```python
from build123d import *

# Parameters (mm, degrees)
BOSS_EXTRUDE1_DEPTH   = 6.35
F_4_40_TAPPED_HOLE1_D = 2.2606
SKETCH8_R             = 2.38125
CUT_EXTRUDE1_DEPTH    = 6.35
SKETCH9_R             = 1.4732
CUT_EXTRUDE2_DEPTH    = 14.088396137
SKETCH10_R            = 1.4732
CUT_EXTRUDE3_DEPTH    = 15.889903931
CHAMFER1_SIZE         = 1.778
CHAMFER1_SIZE_2       = 1.54559182


with BuildPart() as part:
    # Sketch1 → Boss-Extrude1 (new body)
    with BuildSketch(Plane(origin=(0, 0, 0), x_dir=(1, 0, 0), z_dir=(0, 1, 0))):
        with BuildLine():
            Line((-2.487063329, -0.254), (-9.521612731, -0.254))
            ThreePointArc((-9.521612731, -0.254), (0, -9.525), (9.521612731, -0.254))
            Line((9.521612731, -0.254), (2.487063329, -0.254))
            ThreePointArc((2.487063329, -0.254), (0, -2.5), (-2.487063329, -0.254))
        make_face()
    extrude(amount=BOSS_EXTRUDE1_DEPTH)

    # #4-40 Tapped Hole1 (through all)
    with Locations(Plane(origin=(0, 0, 0.254), x_dir=(-1, 0, 0), z_dir=(0, 0, -1))):
        with Locations((6.35, 3.175)):
            Hole(F_4_40_TAPPED_HOLE1_D / 2)

    # Sketch8 → Cut-Extrude1 (cut)
    with BuildSketch(Plane.XY.offset(9.525)):
        with Locations((6.35, 3.175)):
            Circle(SKETCH8_R)
    extrude(amount=-CUT_EXTRUDE1_DEPTH, mode=Mode.SUBTRACT)

    # Sketch9 → Cut-Extrude2 (cut, through all)
    with BuildSketch(Plane.XY.offset(3.175)):
        with Locations((6.35, 3.175)):
            Circle(SKETCH9_R)
    extrude(amount=-CUT_EXTRUDE2_DEPTH, mode=Mode.SUBTRACT)

    # Sketch10 → Cut-Extrude3 (cut, through all)
    with BuildSketch(Plane(origin=(0, 6.35, 0), x_dir=(1, 0, 0), z_dir=(0, 1, 0))):
        with Locations(Location((0, -6.2992, 0), (0, 0, 270))):
            Circle(SKETCH10_R)
    extrude(amount=-CUT_EXTRUDE3_DEPTH, mode=Mode.SUBTRACT)

    # Chamfer1
    # the kernel refuses this chamfer: 1.778, 1.54559182 mm, written as the material it takes off along each edge
    with BuildSketch(Plane(origin=(0, 6.35, 6.2992), x_dir=(0, 0, 1), z_dir=(-1, 0, 0))) as chamfer1_piece_1:
        Polygon((1.4732 + CHAMFER1_SIZE, 0), (1.4732, -CHAMFER1_SIZE_2), (1.4732, 0), align=None)
    revolve(axis=Axis((0, 6.35, 6.2992), (0, 1, 0)), mode=Mode.SUBTRACT)


solid = part.part
```
Input: part model. Units: mm. Frame: model coordinates. A direction names the side the tool comes from. Give positions to 0.01 mm unless a question says otherwise; leave off trailing zeros. Order: outer loops, then holes, each group sorted by start corner. A loop starts at its lowest first (then second) coordinate and runs counter-clockwise, first axis right, second up.
1. Section C-C on x = -6.35. Return the cut outline in (y, z), and give its area (3 significant figures).
Derived:
outline: (0, 0.25) - (2.04, 0.25) - (2.04, 7.1) - (0, 7.1) - close; (4.31, 0.25) - (6.35, 0.25) - (6.35, 7.1) - (4.31, 7.1) - close
area: 28.0 mm2
2. Reachability of faces 1 (the flat face through (-0.1, 6.35, 2.8)), 2 (the flat face through (5, 2, 3.175)) from +Z, -Z, +X, -X, +Y, -Y: full face, straight path, thin tool, end or side. Return the list, or none.
Derived:
face 1: +Z, -Z, +X, -X, +Y
face 2: +Z
3. Material intervals for L1, parallel to X at y = 2.25, z = 1.5; L2, parallel to Y at x = -6.35, z = 2.75; L3, parallel to X at y = 3.75, z = 3.5, sorted ascending.
Derived:
L1: x = -9.41 to -7, -5.7 to -2, 2 to 5.2, 7.5 to 9.41
L2: y = 0 to 2.04, 4.31 to 6.35
L3: x = -8.86 to -7.32, -5.38 to 4.04, 8.66 to 8.86
4. Section D-D on y = 1. Return the cut outline in (x, z) (3 decimals), and give its area (3 significant figures).
Derived:
outline: (-9.522, 0.254) - (-2.487, 0.254) arc R2.5 cw to (2.487, 0.254) - (9.522, 0.254) arc R9.525 ccw to (7.319, 6.095) - (7.319, 3.175) - (5.381, 3.175) - (5.381, 7.86) arc R9.525 ccw to start; hole circle Ø2.946 at (0, 6.299)
area: 115 mm2
5. Mould query, pull axis Y, two halves, no side actions, for faces 3 (the cylindrical face through (5.18, 2.28, 1.73)), 4 (the cylindrical face through (3.97, 3.28, 5.35)), 5 (the flat face through (0, 0, 4)), 6 (the conical face through (0, 5, 8)). Classes: released by +Y, released by -Y, zero draft, split by the parting line, or undercut.
Derived:
face 3: undercut
face 4: undercut
face 5: released by -Y
face 6: released by +Y
6. Section B-B on y = 2.75. Give the number of separate pieces and of enclosed holes in the cut face, and give its area (3 significant figures).
Derived:
separate pieces: 3
enclosed holes: 1
area: 82.6 mm2
7. Section A-A on z = 2. Return the cut outline in (x, y) (3 decimals), and give its area (3 significant figures).
Derived:
outline: (-9.313, 0) - (-1.5, 0) - (-1.5, 6.35) - (-9.313, 6.35) - close; (1.5, 0) - (9.313, 0) - (9.313, 6.35) - (1.5, 6.35) - close; hole circle Ø2.261 at (-6.35, 3.175); hole circle Ø2.946 at (6.35, 3.175)
area: 88.4 mm2
8. Pin query (flat end, axial travel): pin 1 (1.8 mm diameter, centred on x = -6.35, y = 3.175, fed in from -Z); pin 2 (4 mm diameter, centred on x = 0, z = 6.3, fed in from -Y); pin 3 (1.5 mm diameter, centred on y = 4, z = 5, fed in from +X). Return the tip coordinate at first contact, or that it passes through.
Derived:
pin 1: passes through
pin 2: stops at y = 0
pin 3: stops at x = 8.51
